Could you check a few things on this model? Use its own coordinates, in mm. A direction names the side the tool comes from. Coordinates: 2 decimals unless noted, no trailing zeros. Write each loop counter-clockwise with the first axis right and the second up, starting at its lowest first coordinate (ties: lowest second). Pieces come first, ordered by that corner, then holes. Notation, with made-up numbers: (44, -2) - (79, -2) arc R3 cw to (79, 3) - close; hole circle Ø5 at (70.5, -12.75). An arc over 180 degrees is marked (long way). Answer as a JSON object with one key per item and string values. Group by question number.
1) If we section it at D-D (z = -10.25): Write out the boundary of the cut face in (x, y), plus the area to 3 significant figures.
2) If we section it at C-C (z = 0.75): Write out the boundary of the cut face in (x, y).
3) On a 3-axis mill with a long thin cutter (end or side, diameter ignored), from which of +Z, -Z, +X, -X, +Y, -Y can I reach the whole of each face in a straight line? I mean faces 1 (the flat face through (-8.25, -4, 0)), 2 (the flat face through (-7, -2, 0)), 3 (the flat face through (0, -5, -9.5)). Say none if no direction works.
4) We'd pull the mould along Z, two halves only. Please class faces 4 (the flat face through (-9, -1.8, 1)), 5 (the flat face through (7, -2, 0)), 6 (the flat face through (0, -4, -13.8)): released by +Z, released by -Z, zero draft, split by the parting line, or undercut.
5) Will these pins go through, and if not, where does the flat tip stop? pin 1 Ø1.6 at (y, z) = (-4.5, -1) entering from +X; pin 2 Ø2 at (y, z) = (-5, 2) entering from -X; pin 3 Ø1 at (x, y) = (-0.5, -4) entering from -Z.
6) If we section it at B-B (y = -4.15): Write out the boundary of the cut face in (x, z), plus the area to 3 significant figures.
7) Please list where these lines run through material, in increasing order: line 1 along X through (y, z) = (-0.2, -7.75); line 2 along Z through (x, y) = (-0.75, -0.3); line 3 along X through (y, z) = (-3.3, -6).
8) If we section it at A-A (x = -1.75): Write out the boundary of the cut face in (y, z).
```python
from build123d import *

# Parameters (mm, degrees)
F0_W     = 22
F0_H     = 30
F1_DEPTH = 1.8
F2_W     = 16.5
F2_H     = 27.6
F3_DEPTH = 3.8
F4_W     = 12.9
F4_H     = 19
F5_DEPTH = 25
F6_W     = 14
F6_H     = 22
F7_DEPTH = 3.6


with BuildPart() as f1:
    # F0 (on Front) → F1 (new body)
    with BuildSketch(Plane.XZ):
        Rectangle(F0_W, F0_H)
    extrude(amount=F1_DEPTH)

    # F2 (on face) → F3 (join)
    with BuildSketch(Plane.XZ.offset(1.8)):
        Rectangle(F2_W, F2_H)
    extrude(amount=F3_DEPTH)

    # F4 (on face) → F5 (cut)
    with BuildSketch(Plane.XZ.offset(5.6)):
        Rectangle(F4_W, F4_H)
    extrude(amount=-F5_DEPTH, mode=Mode.SUBTRACT)

    # F6 (on face) → F7 (cut)
    with BuildSketch(Plane(origin=(0, 0, 0), x_dir=(-1, 0, 0), z_dir=(0, 1, 0))):
        Rectangle(F6_W, F6_H)
    extrude(amount=-F7_DEPTH, mode=Mode.SUBTRACT)


solid = f1.part
```
Here are the results:
{
 "1": {"outline": "(-11, -1.8) - (-8.25, -1.8) - (-8.25, -5.6) - (8.25, -5.6) - (8.25, -1.8) - (11, -1.8) - (11, 0) - (7, 0) - (7, -3.6) - (-7, -3.6) - (-7, 0) - (-11, 0) - close", "area": "51.9 mm²"},
 "2": {"outline": "(-11, -1.8) - (-8.25, -1.8) - (-8.25, -5.6) - (-6.45, -5.6) - (-6.45, -3.6) - (-7, -3.6) - (-7, 0) - (-11, 0) - close; (6.45, -5.6) - (8.25, -5.6) - (8.25, -1.8) - (11, -1.8) - (11, 0) - (7, 0) - (7, -3.6) - (6.45, -3.6) - close"},
 "3": {"face 1": "+Z, -Z, -X, -Y", "face 2": "+Y", "face 3": "+Y, -Y"},
 "4": {"face 4": "zero draft", "face 5": "undercut", "face 6": "released by -Z"},
 "5": {"pin 1": "stops at x = 8.25", "pin 2": "stops at x = -8.25", "pin 3": "stops at z = -13.8"},
 "6": {"outline": "(-8.25, -13.8) - (8.25, -13.8) - (8.25, 13.8) - (-8.25, 13.8) - close; hole (-6.45, -9.5) - (6.45, -9.5) - (6.45, 9.5) - (-6.45, 9.5) - close", "area": "210 mm²"},
 "7": {"line 1": "x = -11 to -7, 7 to 11", "line 2": "z = -15 to -11, 11 to 15", "line 3": "x = -8.25 to -7, 7 to 8.25"},
 "8": {"outline": "(-5.6, -13.8) - (-1.8, -13.8) - (-1.8, -15) - (0, -15) - (0, -11) - (-3.6, -11) - (-3.6, -9.5) - (-5.6, -9.5) - close; (-5.6, 9.5) - (-3.6, 9.5) - (-3.6, 11) - (0, 11) - (0, 15) - (-1.8, 15) - (-1.8, 13.8) - (-5.6, 13.8) - close"}
}
